Geometry check sheet. Reference: the model listing, model coordinates, mm. A direction names the side the tool comes from. Give positions to 0.01 mm unless a question says otherwise; leave off trailing zeros. Loops run counter-clockwise (first coordinate to the right, second up) from the corner with the lowest first, then second, coordinate; pieces in that order, holes last. Notation, with made-up numbers: (-11.75, -3.75) - (20.25, -3.75) arc R22 ccw to (20.25, 10.25) - close; hole circle Ø4 at (-12, 54). An arc over 180 degrees is marked (long way). Use a Markdown table: item, result. Add a question column.
1. Depth check by flat-ended pin: P1, Ø0.9, axis at y = 24, z = 6, coming from the -X side; P2, Ø0.6, axis at y = 22.5, z = 30, coming from the +X side; P3, Ø0.5, axis at x = -1.5, y = 21, coming from the +Z side. Enter the tip coordinate at first touch or a pass-through.
2. Material ranges on L1, parallel to X at y = 25.3, z = 27.25; L2, parallel to Y at x = 0, z = 41.5; L3, parallel to Z at x = 7.5, y = -14.5, recorded low to high.
3. Cross-section at D-D on z = 6. Enter the section's corners in (x, y).
4. Draft check along Y on faces 1 (the flat face through (2.75, 23, 6)), 2 (the cylindrical face through (-0.08, -16.65, 36.14)), 3 (the cylindrical face through (0.806, 11.415, 40.635)). Enter one of: pulls with the +Y half, pulls with the -Y half, needs draft (parallel to the pull), parting line crosses it, or undercut.
5. Cross-section at C-C on z = 36. Enter the section's corners in (x, y), and give its area (3 significant figures).
6. Cross-section at A-A on y = -25.3. Enter the section's corners in (x, z), and give its area (3 significant figures).
7. Cross-section at B-B on z = 19. Enter the section's corners in (x, y), and give its area (3 significant figures).
8. Set-up check for faces 4 (the flat face through (9, -4, 36)), 5 (the flat face through (0, -20.15, 32)), 6 (the flat face through (0, -20.15, 13)), 7 (the flat face through (0, 26.8, 28)): record each of +Z, -Z, +X, -X, +Y, -Y from which the full face is reachable in a straight line by a thin tool's end or side.
from build123d import *

# Parameters (mm, degrees)
SKETCH_W        = 20
SKETCH_H        = 40.3
PAD_DEPTH       = 26.6
SKETCH001_W     = 20
SKETCH001_H     = 53.6
PAD001_DEPTH    = 2.5
SKETCH002_W     = 20
SKETCH002_H     = 40.3
PAD002_DEPTH    = 6
PAD003_DEPTH    = 2.5
SKETCH004_R     = 6.5
PAD004_DEPTH    = 1
SKETCH005_R     = 5.5
PAD005_DEPTH    = 0.5
SKETCH006_R     = 3
PAD006_DEPTH    = 4
SKETCH007_R     = 1.5
POCKET_DEPTH    = 5
SKETCH008_R     = 2.25
POCKET001_DEPTH = 5
SKETCH009_W     = 1
SKETCH009_H     = 6.65
PAD007_DEPTH    = 2
POCKET002_DEPTH = 1
FILLET_R        = 0.4
SKETCH011_W     = 6.5
SKETCH011_H     = 4
PAD008_DEPTH    = 1
SKETCH012_W     = 5.5
SKETCH012_H     = 3
PAD009_DEPTH    = 4
SKETCH013_R     = 0.75
PAD010_DEPTH    = 10


with BuildPart() as part:
    # Sketch → Pad (new body)
    with BuildSketch(Plane.XY):
        Rectangle(SKETCH_W, SKETCH_H)
    extrude(amount=PAD_DEPTH)

    # Sketch001 (on Face6 of Pad) → Pad001 (join)
    with BuildSketch(Plane.XY.offset(26.6)):
        Rectangle(SKETCH001_W, SKETCH001_H)
    extrude(amount=PAD001_DEPTH)

    # Sketch002 (on Face5 of Pad001) → Pad002 (join)
    with BuildSketch(Plane.XY.offset(29.1)):
        Rectangle(SKETCH002_W, SKETCH002_H)
    extrude(amount=PAD002_DEPTH)

    # Sketch003 (on Face18 of Pad002) → Pad003 (join)
    with BuildSketch(Plane.XY.offset(35.1)):
        with BuildLine():
            ThreePointArc((9, 7.108619), (0, 19.65), (-9, 7.108619))
            Line((-9, 7.108619), (-9, -14.15))
            Line((-9, -14.15), (-5, -14.15))
            ThreePointArc((-5, -14.15), (0, -16.65), (5, -14.15))
            Line((5, -14.15), (9, -14.15))
            Line((9, -14.15), (9, 7.108619))
        make_face()
    extrude(amount=PAD003_DEPTH)

    # Sketch004 (on Face25 of Pad003) → Pad004 (join)
    with BuildSketch(Plane.XY.offset(37.6)):
        with Locations((0, 10.15)):
            Circle(SKETCH004_R)
    extrude(amount=PAD004_DEPTH)

    # Sketch005 (on Face27 of Pad004) → Pad005 (join)
    with BuildSketch(Plane.XY.offset(38.6)):
        with Locations((0, 10.15)):
            Circle(SKETCH005_R)
    extrude(amount=PAD005_DEPTH)

    # Sketch006 (on Face29 of Pad005) → Pad006 (join)
    with BuildSketch(Plane.XY.offset(39.1)):
        with Locations((0, 10.15)):
            Circle(SKETCH006_R)
    extrude(amount=PAD006_DEPTH)

    # Sketch007 (on Face31 of Pad006) → Pocket (cut)
    with BuildSketch(Plane.XY.offset(43.1)):
        with Locations((0, 10.15)):
            Circle(SKETCH007_R)
    extrude(amount=-POCKET_DEPTH, mode=Mode.SUBTRACT)

    # Sketch008 (on Face5 of Pocket) → Pocket001 (cut)
    with BuildSketch(Plane.XY.offset(29.1)):
        with Locations((-4.911566, 25.3)):
            Circle(SKETCH008_R)
        with Locations((4.911566, 25.3)):
            Circle(SKETCH008_R)
        with Locations((-4.911566, -25.3)):
            Circle(SKETCH008_R)
        with Locations((4.911566, -25.3)):
            Circle(SKETCH008_R)
    extrude(amount=-POCKET001_DEPTH, mode=Mode.SUBTRACT)

    # Sketch009 (on Face4 of Pocket001) → Pad007 (join)
    with BuildSketch(Plane.XY.offset(29.1)):
        with Locations((0, 23.475)):
            Rectangle(SKETCH009_W, SKETCH009_H)
        with Locations((0, -23.475)):
            Rectangle(SKETCH009_W, SKETCH009_H)
    extrude(amount=PAD007_DEPTH)

    # Sketch010 (on Face28 of Pad007) → Pocket002 (cut)
    with BuildSketch(Plane.YZ.offset(0.5)):
        Polygon((-26.8, 29.1), (-26.8, 31.1), (-20.15, 31.1), align=None)
        Polygon((20.15, 31.1), (26.8, 31.1), (26.8, 29.1), align=None)
    extrude(amount=-POCKET002_DEPTH, mode=Mode.SUBTRACT)

    # Fillet
    fillet_edges = [part.edges().sort_by_distance(p)[0] for p in [
        (10, -20.15, 13.3),
        (-10, -20.15, 13.3),
        (10, 20.15, 13.3),
        (-10, 20.15, 13.3),
        (-10, 20.15, 32.1),
        (10, 20.15, 32.1),
        (-10, -20.15, 32.1),
        (10, -20.15, 32.1),
        (-10, 0, 35.1),
        (0, -20.15, 35.1),
        (10, 0, 35.1),
        (0, 20.15, 35.1),
        (10, 26.8, 27.85),
        (-10, 26.8, 27.85),
        (-10, -26.8, 27.85),
        (10, -26.8, 27.85),
        (0, 19.65, 37.6),
        (-9, -3.520691, 37.6),
        (-7, -14.15, 37.6),
        (0, -16.65, 37.6),
        (7, -14.15, 37.6),
        (9, -3.520691, 37.6),
        (-3, 10.15, 43.1),
        (0, 20.15, 0),
        (10, 0, 0),
        (0, -20.15, 0),
        (-10, 0, 0),
    ]]
    fillet(fillet_edges, radius=FILLET_R)

    # Sketch011 (on Face50 of Fillet) → Pad008 (join)
    with BuildSketch(Plane(origin=(0, 20.15, 0), x_dir=(-1, 0, 0), z_dir=(0, 1, 0))):
        with Locations((0, 6)):
            Rectangle(SKETCH011_W, SKETCH011_H)
    extrude(amount=PAD008_DEPTH)

    # Sketch012 (on Face77 of Pad008) → Pad009 (join)
    with BuildSketch(Plane(origin=(0, 21.15, 0), x_dir=(-1, 0, 0), z_dir=(0, 1, 0))):
        with Locations((0, 6)):
            Rectangle(SKETCH012_W, SKETCH012_H)
    extrude(amount=PAD009_DEPTH)

    # Sketch013 (on Face89 of Pad009) → Pad010 (join)
    with BuildSketch(Plane(origin=(0, 25.15, 0), x_dir=(-1, 0, 0), z_dir=(0, 1, 0))):
        with Locations((-1.55, 6)):
            Circle(SKETCH013_R)
        with Locations((0, 6)):
            Circle(SKETCH013_R)
        with Locations((1.55, 6)):
            Circle(SKETCH013_R)
    extrude(amount=PAD010_DEPTH)


solid = part.part
Values found:
| question | item | result |
|---|---|---|
| 1 | P1 | stops at x = -2.75 |
| 1 | P2 | stops at x = 0.5 |
| 1 | P3 | stops at z = 29.1 |
| 2 | L1 | x = -10 to -7.16, -2.66 to 2.66, 7.16 to 10 |
| 2 | L2 | y = 7.15 to 8.65, 11.65 to 13.15 |
| 2 | L3 | z = 0 to 35.1 |
| 3 | outline | (-10, -19.75) arc R0.4 ccw to (-9.6, -20.15) - (9.6, -20.15) arc R0.4 ccw to (10, -19.75) - (10, 19.75) arc R0.4 ccw to (9.6, 20.15) - (3.25, 20.15) - (3.25, 21.15) - (2.75, 21.15) - (2.75, 25.15) - (2.3, 25.15) - (2.3, 35.15) - (0.8, 35.15) - (0.8, 25.15) - (0.75, 25.15) - (0.75, 35.15) - (-0.75, 35.15) - (-0.75, 25.15) - (-0.8, 25.15) - (-0.8, 35.15) - (-2.3, 35.15) - (-2.3, 25.15) - (-2.75, 25.15) - (-2.75, 21.15) - (-3.25, 21.15) - (-3.25, 20.15) - (-9.6, 20.15) arc R0.4 ccw to (-10, 19.75) - close |
| 4 | face 1 | needs draft |
| 4 | face 2 | pulls with the -Y half |
| 4 | face 3 | undercut |
| 5 | outline | (-9, -14.15) - (-5, -14.15) arc R6.25 ccw to (5, -14.15) - (9, -14.15) - (9, 7.11) arc R9.5 ccw (long way) to (-9, 7.11) - close |
| 5 | area | 599 mm2 |
| 6 | outline | (-10, 26.6) - (-7.16, 26.6) - (-7.16, 29.1) - (-10, 29.1) - close; (-2.66, 26.6) - (2.66, 26.6) - (2.66, 29.1) - (0.5, 29.1) - (0.5, 29.55) - (-0.5, 29.55) - (-0.5, 29.1) - (-2.66, 29.1) - close; (7.16, 26.6) - (10, 26.6) - (10, 29.1) - (7.16, 29.1) - close |
| 6 | area | 28.0 mm2 |
| 7 | outline | (-10, -19.75) arc R0.4 ccw to (-9.6, -20.15) - (9.6, -20.15) arc R0.4 ccw to (10, -19.75) - (10, 19.75) arc R0.4 ccw to (9.6, 20.15) - (-9.6, 20.15) arc R0.4 ccw to (-10, 19.75) - close |
| 7 | area | 806 mm2 |
| 8 | face 4 | +Z, +X, -Y |
| 8 | face 5 | +Z, -Y |
| 8 | face 6 | -Z, +X, -X, -Y |
| 8 | face 7 | +Z, +X, -X, +Y |
